Build history of the part. All positions in model axes, mm. Face numbers are marked on the shaded views. A direction names the side the tool comes from. Coordinates: 2 decimals unless noted, no trailing zeros. Order: outer loops, then holes, each group sorted by start corner. A loop starts at its lowest first (then second) coordinate and runs counter-clockwise, first axis right, second up. Notation, with made-up numbers: M -21,61.5 L -16,61.5 A30 ccw -16,87.5 Z; hole C 13.25,-23 d3. An arc over 180 degrees is marked long. Use a Markdown table: item, result. Add a question column.
from build123d import *

# Parameters (mm, degrees)
ENL_V_MAT_EXTRU_1_DEPTH      = 750.28036314
ENL_V_MAT_EXTRU_1_DEPTH_BACK = 750.28036314
ENL_V_MAT_EXTRU_2_DEPTH      = 745.848977981
ESQUISSE5_R                  = 30
BOSS_EXTRU_1_DEPTH           = 90
CHANFREIN2_SIZE              = 5


with BuildPart() as part:
    # Esquisse1 → Révolution1 (revolve)
    with BuildSketch(Plane.XY, mode=Mode.PRIVATE) as r_volution1_sk:
        Polygon((4.713461336, 0), (344.713461336, 0), (384.713461336, 70), (704.713461336, 70), (704.713461336, 180), (664.713461336, 180), (664.713461336, 90), (634.713461336, 90), (634.713461336, 100), (184.713461336, 100), (184.713461336, 60), (4.713461336, 60), align=None)
    revolve(r_volution1_sk.sketch.rotate(Axis((4.713461336, 0, 0), (1, 0, 0)), 180), axis=Axis((4.713461336, 0, 0), (1, 0, 0)))

    # Esquisse2 → Enlèv. mat.-Extru.1 (cut, two sides: drawn at the far end of the back side and taken through both)
    with BuildSketch(Plane.XY.offset(-ENL_V_MAT_EXTRU_1_DEPTH_BACK)):
        with BuildLine():
            Line((424.713461336, 100), (544.713461336, 100))
            Line((544.713461336, 100), (544.713461336, 55))
            ThreePointArc((544.713461336, 55), (540.320063053, 44.393398282), (529.713461336, 40))
            Line((529.713461336, 40), (439.713461336, 40))
            ThreePointArc((439.713461336, 40), (429.106859618, 44.393398282), (424.713461336, 55))
            Line((424.713461336, 55), (424.713461336, 100))
        make_face()
    extrude(amount=ENL_V_MAT_EXTRU_1_DEPTH + ENL_V_MAT_EXTRU_1_DEPTH_BACK, mode=Mode.SUBTRACT)

    # Esquisse4 → Enlèv. mat.-Extru.2 (cut, through all)
    with BuildSketch(Plane(origin=(704.713461336, 0, 0), x_dir=(0, 0, -1), z_dir=(1, 0, 0))):
        with BuildLine():
            Line((-120, 0), (-70, 165.831239518))
            ThreePointArc((-70, 165.831239518), (-150, 99.498743711), (-180, 0))
            Line((-180, 0), (-120, 0))
        make_face()
        with BuildLine():
            ThreePointArc((180, 0), (150, 99.498743711), (70, 165.831239518))
            Line((70, 165.831239518), (120, 0))
            Line((120, 0), (180, 0))
        make_face()
    extrude(amount=-ENL_V_MAT_EXTRU_2_DEPTH, mode=Mode.SUBTRACT)

    # Esquisse5 → Boss.-Extru.1 (add)
    with BuildSketch(Plane(origin=(704.713461336, 0, 0), x_dir=(0, 0, -1), z_dir=(1, 0, 0))):
        with Locations(Location((0, 125, 0), (0, 0, 270))):
            Circle(ESQUISSE5_R)
    extrude(amount=BOSS_EXTRU_1_DEPTH)

    # Chanfrein2
    chanfrein2_edges = [part.edges().sort_by_distance(p)[0] for p in [
        (704.713461336, 155, 0),
        (704.713461336, -180, 0),
    ]]
    chamfer(chanfrein2_edges, length=CHANFREIN2_SIZE)


solid = part.part
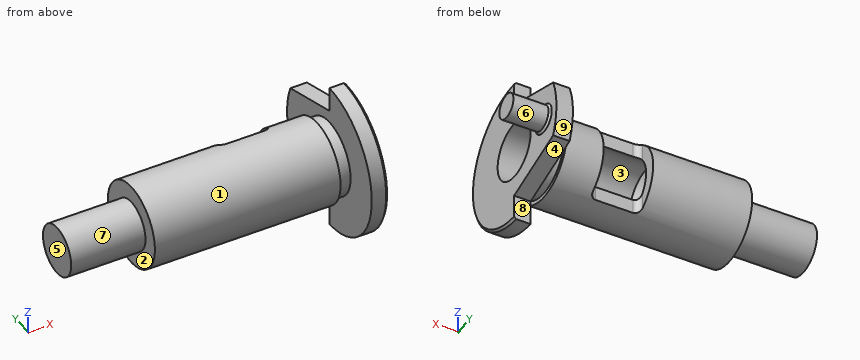
(1) Drop flat-ended pins along their axis: P1, Ø13.5, axis at y = 72.5, z = -15.5, coming from the -X side; P2, Ø12, axis at x = 687.5, z = 165, coming from the +Y side; P3, Ø1, axis at y = -25.5, z = 76, coming from the +X side. Give the stop position or say it passes through.
(2) Slice it at D-D on x = 131.5. Give the cut face in (y, z).
(3) Mould opens along Z. For the marked faces 1, 2, 3 and 4 say: released by +Z, released by -Z, zero draft, split by the parting line, or undercut.
(4) Slice it at B-B on y = 125. Give the cut face in (x, z).
(5) Slice it at C-C on x = 450. Give the cut face in (y, z).
(6) Which spindle directions (+Z, -Z, +X, -X, +Y, -Y) get a long thin tool onto all of the face, cutting with end or side? Do the marked faces 5, 6, 7, 8 and 9. Say none if no direction does.
(7) Drill centre lines: line 1 along X through (y, z) = (70.5, -69.5); line 2 along Z through (x, y) = (584, 0); line 3 along X through (y, z) = (-8.5, -92.5). Where is each one in solid material? Low to high. Write a range as from..to.
(8) Slice it at A-A on x = 672.5. Give the cut face in (y, z).
Solutions:
| question | item | result |
|---|---|---|
| 1 | P1 | x = 184.71 |
| 1 | P2 | y = 0 |
| 1 | P3 | x = 704.71 |
| 2 | outline | C 0,0 d120 |
| 3 | face 1 | split by the parting line |
| 3 | face 2 | zero draft |
| 3 | face 3 | undercut |
| 3 | face 4 | released by -Z |
| 4 | outline | M 664.71,-82.31 L 704.71,-82.31 L 704.71,-35 L 709.71,-30 L 794.71,-30 L 794.71,30 L 709.71,30 L 704.71,35 L 704.71,82.31 L 664.71,82.31 Z |
| 5 | outline | M 40,-91.65 L 40,-57.45 A70 cw long 40,57.45 L 40,91.65 A100 ccw long Z |
| 6 | face 5 | +Z, -Z, -X, +Y, -Y |
| 6 | face 6 | +X |
| 6 | face 7 | -X |
| 6 | face 8 | -Z, +X, -X, +Y |
| 6 | face 9 | +X, -X, +Y |
| 7 | line 1 | 184.71..424.71, 544.71..634.71, 664.71..704.71 |
| 7 | line 2 | -100..-70, 70..100 |
| 7 | line 3 | 184.71..634.71, 664.71..704.71 |
| 8 | outline | M 0,-180 L 0,-120 L 165.83,-70 A180 ccw 165.83,70 L 0,120 L 0,180 A180 ccw Z; hole C 0,0 d140 |
